```python
from build123d import *

# Parameters (mm, degrees)
SALIENTE_EXTRUIR1_DEPTH                              = 15
CROQUIS2_R                                           = 60
SALIENTE_EXTRUIR2_DEPTH                              = 5
REFRENTADO_PARA_TORNILLO_CON_CABEZA_TRON_D           = 3.4
REFRENTADO_PARA_TORNILLO_CON_CABEZA_TRON_CBORE_D     = 7
REFRENTADO_PARA_TORNILLO_CON_CABEZA_TRON_CBORE_DEPTH = 2.4


with BuildPart() as part:
    # Croquis1 → Saliente-Extruir1 (new body)
    with BuildSketch(Plane.XY):
        with BuildLine():
            Line((-15, -49.849774322), (-15, -54.083269132))
            ThreePointArc((-15, -54.083269132), (-16.245307044, -56.516590449), (-18.947368421, -56.929756981))
            ThreePointArc((-18.947368421, -56.929756981), (0, 60), (18.947368421, -56.929756981))
            ThreePointArc((18.947368421, -56.929756981), (16.245307044, -56.516590449), (15, -54.083269132))
            Line((15, -54.083269132), (15, -49.849774322))
            ThreePointArc((15, -49.849774322), (15.544739955, -48.125912926), (16.981132075, -47.028088983))
            ThreePointArc((16.981132075, -47.028088983), (0, 50), (-16.981132075, -47.028088983))
            ThreePointArc((-16.981132075, -47.028088983), (-15.544739955, -48.125912926), (-15, -49.849774322))
        make_face()
    extrude(amount=SALIENTE_EXTRUIR1_DEPTH)

    # Croquis2 → Saliente-Extruir2 (add)
    with BuildSketch(Plane.XY.offset(15)):
        with Locations(Location((0, 0, 0), (0, 0, 251.591519829))):
            Circle(CROQUIS2_R)
    extrude(amount=SALIENTE_EXTRUIR2_DEPTH)

    # Refrentado para tornillo con cabeza troncocónica de M31 (through all)
    with Locations(Plane.XY.offset(20)):
        with Locations((-21.04758878, 50.813374288), (21.04758878, 50.813374288), (50.813374288, 21.04758878), (50.813374288, -21.04758878), (21.04758878, -50.813374288), (-21.04758878, -50.813374288), (-50.813374288, -21.04758878), (-50.813374288, 21.04758878)):
            CounterBoreHole(REFRENTADO_PARA_TORNILLO_CON_CABEZA_TRON_D / 2, REFRENTADO_PARA_TORNILLO_CON_CABEZA_TRON_CBORE_D / 2, REFRENTADO_PARA_TORNILLO_CON_CABEZA_TRON_CBORE_DEPTH)


solid = part.part
```
The model under review builds one solid part; all positions refer to its coordinate system, in mm. A direction names the side the tool comes from. Round coordinates to 2 decimals unless told otherwise and drop trailing zeros. Loops run counter-clockwise (first coordinate to the right, second up) from the corner with the lowest first, then second, coordinate; pieces in that order, holes last. Notation, with made-up numbers: (13, 13) - (25, 13) arc R16 cw to (25, 29) - close; hole circle Ø2 at (63, -21.75). An arc over 180 degrees is marked (long way). Use a Markdown table: item, result. Add a question column.
Q1. Add section D-D (x = 33.5). State the section outline as (y, z) points.
Q2. Machinability: for faces 3 (the face through (15, -52, 7)), 4 (the face through (15.53, -48.15, 7.4)), 5 (the face through (-22, 49, 17.6)), 6 (the face through (22.397, -51.848, 8.677)), which of the approach directions +Z, -Z, +X, -X, +Y, -Y give a long, thin tool a straight path to every point of the face, cutting with its end or side? Answer none if there is none.
Q3. Add section B-B (x = 0). State the section outline as (y, z) points.
Q4. For probe 1 along X at (y, z) = (-49.5, 19); probe 2 along Y at (x, z) = (-52, 12.25); probe 3 along Z at (x, y) = (-20, 10), list the stretches that pass through material, from the lowest coordinate up.
Q5. The part is to be moulded in two halves that separate along X. For faces 1 (the face through (-19.166, 53.765, 18.817)), 2 (the face through (9.2, 49.4, 0)), say which applies: pulls with the +X half, pulls with the -X half, needs draft (parallel to the pull), parting line crosses it, or undercut.
Q6. Add section C-C (z = 7). State how many separate pieces and enclosed holes the cut face has, plus the area to 3 significant figures.
Q7. Insertion check: pin 1 Ø10 at (x, z) = (-6, 8.5) entering from +Y; pin 2 Ø4.5 at (x, y) = (-50.81, -21.05) entering from +Z; pin 3 Ø10 at (x, y) = (14, 22) entering from -Z. Each pin has a flat end and moves straight along its axis. Give the tip position at first contact, or say it passes through.
Q8. Add section A-A (y = 0). State the section outline as (x, z) points.
Worked answers:
| question | item | result |
|---|---|---|
| 1 | outline | (-49.78, 0) - (-37.12, 0) - (-37.12, 15) - (37.12, 15) - (37.12, 0) - (49.78, 0) - (49.78, 20) - (-49.78, 20) - close |
| 2 | face 3 | -Z, -Y |
| 2 | face 4 | -Z |
| 2 | face 5 | +Z |
| 2 | face 6 | +Z, -Z |
| 3 | outline | (-60, 15) - (50, 15) - (50, 0) - (60, 0) - (60, 20) - (-60, 20) - close |
| 4 | probe 1 | -33.91 to -24.29, -17.8 to 17.8, 24.29 to 33.91 |
| 4 | probe 2 | -29.93 to -22.26, -19.83 to 19.83, 22.26 to 29.93 |
| 4 | probe 3 | 15 to 20 |
| 5 | face 1 | undercut |
| 5 | face 2 | needs draft |
| 6 | separate pieces | 1 |
| 6 | enclosed holes | 8 |
| 6 | area | 3,070 mm² |
| 7 | pin 1 | y = 59.99 |
| 7 | pin 2 | z = 17.6 |
| 7 | pin 3 | z = 15 |
| 8 | outline | (-60, 0) - (-50, 0) - (-50, 15) - (50, 15) - (50, 0) - (60, 0) - (60, 20) - (-60, 20) - close |
